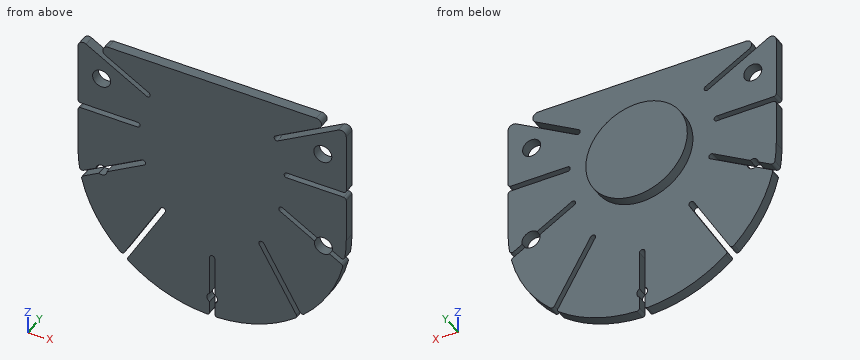
```python
from build123d import *

# Parameters (mm, degrees)
SKETCH2_R                   = 2
BOSS_EXTRUDE1_DEPTH         = 3.81
SKETCH3_R                   = 19.05
BOSS_EXTRUDE2_DEPTH         = 3.81
F_1_4_CLEARANCE_HOLE1_D     = 6.7564
F_1_4_CLEARANCE_HOLE1_DEPTH = 3.81


with BuildPart() as part:
    # Sketch2 → Boss-Extrude1 (new body)
    with BuildSketch(Plane(origin=(0, 0, 0), x_dir=(1, 0, 0), z_dir=(0, 1, 0))):
        with BuildLine():
            Line((40.724728738, 1.878024889), (26.480762114, -6.345733076))
            ThreePointArc((26.480762114, -6.345733076), (25.11473671, -5.979707672), (25.480762114, -4.613682268))
            Line((25.480762114, -4.613682268), (39.724728738, 3.610075697))
            ThreePointArc((39.724728738, 3.610075697), (40.724728738, 5.342126504), (42.724728738, 5.342126504))
            Line((42.724728738, 5.342126504), (48.484388044, 8.667467356))
            ThreePointArc((48.484388044, 8.667467356), (48.902372172, 9.136875637), (48.957702204, 9.762969441))
            ThreePointArc((48.957702204, 9.762969441), (43.570719337, 23.353585317), (34.503184828, 34.821115225))
            ThreePointArc((34.503184828, 34.821115225), (33.67210529, 35.082877041), (32.951211415, 34.593464671))
            Line((32.951211415, 34.593464671), (19.366025404, 11.063232268))
            ThreePointArc((19.366025404, 11.063232268), (18, 10.697206864), (17.633974596, 12.063232268))
            Line((17.633974596, 12.063232268), (31.605824937, 36.263186935))
            ThreePointArc((31.605824937, 36.263186935), (31.722370232, 36.949076207), (31.363324879, 37.544990071))
            ThreePointArc((31.363324879, 37.544990071), (17.573916059, 45.350404511), (2.040567951, 48.478884454))
            ThreePointArc((2.040567951, 48.478884454), (1.307384649, 48.201014802), (1, 47.479707672))
            Line((1, 47.479707672), (1, 43.010935261))
            ThreePointArc((1, 43.010935261), (2, 41.278884454), (1, 39.546833646))
            Line((1, 39.546833646), (1, 24.520292328))
            ThreePointArc((1, 24.520292328), (0, 23.520292328), (-1, 24.520292328))
            Line((-1, 24.520292328), (-1, 39.546833646))
            ThreePointArc((-1, 39.546833646), (-2, 41.278884454), (-1, 43.010935261))
            Line((-1, 43.010935261), (-1, 47.479707672))
            ThreePointArc((-1, 47.479707672), (-1.307384649, 48.201014802), (-2.040567951, 48.478884454))
            ThreePointArc((-2.040567951, 48.478884454), (-17.573916059, 45.350404511), (-31.363324879, 37.544990071))
            ThreePointArc((-31.363324879, 37.544990071), (-31.722370232, 36.949076207), (-31.605824937, 36.263186935))
            Line((-31.605824937, 36.263186935), (-17.633974596, 12.063232268))
            ThreePointArc((-17.633974596, 12.063232268), (-18, 10.697206864), (-19.366025404, 11.063232268))
            Line((-19.366025404, 11.063232268), (-32.951211415, 34.593464671))
            ThreePointArc((-32.951211415, 34.593464671), (-33.67210529, 35.082877041), (-34.503184828, 34.821115225))
            ThreePointArc((-34.503184828, 34.821115225), (-43.570719337, 23.353585317), (-48.957702204, 9.762969441))
            ThreePointArc((-48.957702204, 9.762969441), (-48.902372172, 9.136875637), (-48.484388044, 8.667467356))
            Line((-48.484388044, 8.667467356), (-42.5, 5.212379307))
            ThreePointArc((-42.5, 5.212379307), (-40.5, 5.212379307), (-39.5, 3.4803285))
            Line((-39.5, 3.4803285), (-25.480762114, -4.613682268))
            ThreePointArc((-25.480762114, -4.613682268), (-25.11473671, -5.979707672), (-26.480762114, -6.345733076))
            Line((-26.480762114, -6.345733076), (-40.5, 1.748277692))
            ThreePointArc((-40.5, 1.748277692), (-42.5, 1.748277692), (-43.5, 3.4803285))
            Line((-43.5, 3.4803285), (-48.278351245, 6.239110877))
            ThreePointArc((-48.278351245, 6.239110877), (-49.214035452, 6.273185063), (-49.767770135, 5.518172556))
            ThreePointArc((-49.767770135, 5.518172556), (-50.16676608, 1.878923371), (-50.3, -1.779707672))
            Line((-50.3, -1.779707672), (-50.3, -18.479707672))
            ThreePointArc((-50.3, -18.479707672), (-50.007106781, -19.186814453), (-49.3, -19.479707672))
            Line((-49.3, -19.479707672), (-28, -19.479707672))
            ThreePointArc((-28, -19.479707672), (-27, -20.479707672), (-28, -21.479707672))
            Line((-28, -21.479707672), (-49.3, -21.479707672))
            ThreePointArc((-49.3, -21.479707672), (-50.007106781, -21.772600891), (-50.3, -22.479707672))
            Line((-50.3, -22.479707672), (-50.3, -44.954844537))
            ThreePointArc((-50.3, -44.954844537), (-49.3, -46.686895345), (-47.3, -46.686895345))
            Line((-47.3, -46.686895345), (-24.465777351, -33.503550752))
            ThreePointArc((-24.465777351, -33.503550752), (-23.31681977, -34.116970624), (-23.748711306, -35.345733076))
            Line((-23.748711306, -35.345733076), (-40.033320997, -44.747656864))
            ThreePointArc((-40.033320997, -44.747656864), (-40.965172649, -46.997345762), (-39.033320997, -48.479707672))
            Line((-39.033320997, -48.479707672), (39.033320997, -48.479707672))
            ThreePointArc((39.033320997, -48.479707672), (40.965172649, -46.997345762), (40.033320997, -44.747656864))
            Line((40.033320997, -44.747656864), (23.748711306, -35.345733076))
            ThreePointArc((23.748711306, -35.345733076), (23.31681977, -34.116970624), (24.465777351, -33.503550752))
            Line((24.465777351, -33.503550752), (47.3, -46.686895345))
            ThreePointArc((47.3, -46.686895345), (49.3, -46.686895345), (50.3, -44.954844537))
            Line((50.3, -44.954844537), (50.3, -22.479707672))
            ThreePointArc((50.3, -22.479707672), (50.007106781, -21.772600891), (49.3, -21.479707672))
            Line((49.3, -21.479707672), (28, -21.479707672))
            ThreePointArc((28, -21.479707672), (27, -20.479707672), (28, -19.479707672))
            Line((28, -19.479707672), (49.3, -19.479707672))
            ThreePointArc((49.3, -19.479707672), (50.007106781, -19.186814453), (50.3, -18.479707672))
            Line((50.3, -18.479707672), (50.3, -1.779707672))
            ThreePointArc((50.3, -1.779707672), (50.16676608, 1.878923371), (49.767770135, 5.518172556))
            ThreePointArc((49.767770135, 5.518172556), (49.214035452, 6.273185063), (48.278351245, 6.239110877))
            Line((48.278351245, 6.239110877), (43.724728738, 3.610075697))
            ThreePointArc((43.724728738, 3.610075697), (42.724728738, 1.878024889), (40.724728738, 1.878024889))
        make_face()
        with Locations(Location((-41.5, -34.479707672, 0), (0, 0, 90))):
            Circle(SKETCH2_R, mode=Mode.SUBTRACT)
        with Locations(Location((41.5, -34.479707672, 0), (0, 0, 90))):
            Circle(SKETCH2_R, mode=Mode.SUBTRACT)
    extrude(amount=BOSS_EXTRUDE1_DEPTH)

    # Sketch3 → Boss-Extrude2 (add)
    with BuildSketch(Plane(origin=(0, 3.81, 0), x_dir=(1, 0, 0), z_dir=(0, 1, 0))):
        with Locations(Location((0, -15.459707672, 0), (0, 0, 90))):
            Circle(SKETCH3_R)
    extrude(amount=BOSS_EXTRUDE2_DEPTH)

    # 1/4 Clearance Hole1
    with Locations(Plane(origin=(0, 3.81, 0), x_dir=(1, 0, 0), z_dir=(0, 1, 0))):
        with Locations((41.5, -34.479707672), (41.724728738, 3.610075697), (-41.5, -34.479707672)):
            Hole(F_1_4_CLEARANCE_HOLE1_D / 2, depth=F_1_4_CLEARANCE_HOLE1_DEPTH)


solid = part.part
```
Read the model definition and answer for the solid it produces. Units are mm, in the model's axes. Round coordinates to 2 decimals unless told otherwise and drop trailing zeros. Write each loop counter-clockwise with the first axis right and the second up, starting at its lowest first coordinate (ties: lowest second). Pieces come first, ordered by that corner, then holes. Notation, with made-up numbers: (6.5, -20.5) - (56.5, -20.5) arc R20 cw to (56.5, -14.5) - close; hole circle Ø11 at (75, 11.5). An arc over 180 degrees is marked (long way). Use CSV: the item, a comma, the result in double quotes.
Q1. Each of these flat-tipped pins is pushed along its axis until it touches: pin 1 Ø9 at (x, z) = (41.5, 34.48) entering from +Y; pin 2 Ø1.1 at (y, z) = (1.5, -45) entering from -X; pin 3 Ø1.1 at (x, y) = (-41.5, 2) entering from -Z. Where does it stop, or does it pass through?
Values:
pin 1,"stops at y = 3.81"
pin 2,"stops at x = -19.82"
pin 3,"stops at z = -27.43"
Q2. Find section A-A, the plane z = -20.5. Write down the section's boundary in (x, y).
Values:
outline,"(-45.1, 0) - (-24.81, 0) - (-24.81, 3.81) - (-45.1, 3.81) - close; (-22.5, 0) - (22.5, 0) - (22.5, 3.81) - (-22.5, 3.81) - close; (24.81, 0) - (45.1, 0) - (45.1, 3.81) - (24.81, 3.81) - close"
Q3. Find section B-B, the plane x = 13. Write down the section's boundary in (y, z), then the cut area to 3 significant figures.
Values:
outline,"(0, -46.81) - (3.81, -46.81) - (3.81, 1.53) - (7.62, 1.53) - (7.62, 29.38) - (3.81, 29.38) - (3.81, 48.48) - (0, 48.48) - close"
area,"469 mm²"
Q4. Straight lines are drawn through the part: line 1 along X through (y, z) = (1, 0.5); line 2 along Z through (x, y) = (41.5, 1.6); line 3 along X through (y, z) = (3.75, -0.5). For each, find the intervals that lie inside material, in ascending order.
Values:
line 1,"x = -50.28 to -36.61, -32.61 to 32.61, 36.61 to 50.28"
line 2,"z = -26.64 to -6.98, -0.24 to 19.48, 21.48 to 31.1, 37.86 to 43.34"
line 3,"x = -50.25 to -38.34, -34.34 to 34.34, 38.34 to 40.41, 43.04 to 50.25"
Q5. Find section C-C, the plane x = -12. Write down the section's boundary in (y, z), then the cut area to 3 significant figures.
Values:
outline,"(0, -47.07) - (3.81, -47.07) - (3.81, 0.66) - (7.62, 0.66) - (7.62, 30.26) - (3.81, 30.26) - (3.81, 48.48) - (0, 48.48) - close"
area,"477 mm²"
